```python
from build123d import *

# Parameters (mm, degrees)
SKETCH1_W           = 11.43
SKETCH1_H           = 11.43
BOSS_EXTRUDE1_DEPTH = 6.35
SKETCH3_W           = 6.389415989
SKETCH3_H           = 4.631950103
CUT_EXTRUDE1_DEPTH  = 7.62
SKETCH4_W           = 5.33014865
SKETCH4_H           = 6.972552684
CUT_EXTRUDE2_DEPTH  = 15.24
SKETCH5_W           = 14.938478928
SKETCH5_H           = 9.529491398
BOSS_EXTRUDE2_DEPTH = 6.35


with BuildPart() as part:
    # Sketch1 → Boss-Extrude1 (new body)
    with BuildSketch(Plane(origin=(0, 0, 0), x_dir=(1, 0, 0), z_dir=(0, 1, 0))):
        with Locations((5.715, 5.715)):
            Rectangle(SKETCH1_W, SKETCH1_H)
    extrude(amount=BOSS_EXTRUDE1_DEPTH)

    # Sketch3 → Cut-Extrude1 (cut)
    with BuildSketch(Plane(origin=(0, 0, -11.43), x_dir=(-1, 0, 0), z_dir=(0, 0, -1))):
        with Locations((-8.235292005, 4.034024949)):
            Rectangle(SKETCH3_W, SKETCH3_H)
    extrude(amount=-CUT_EXTRUDE1_DEPTH, mode=Mode.SUBTRACT)

    # Sketch4 → Cut-Extrude2 (cut)
    with BuildSketch(Plane(origin=(0, 1.718049897, 0), x_dir=(1, 0, 0), z_dir=(0, 1, 0))):
        with Locations((5.430693356, 5.379383443)):
            Rectangle(SKETCH4_W, SKETCH4_H)
    extrude(amount=CUT_EXTRUDE2_DEPTH, mode=Mode.SUBTRACT)

    # Sketch5 → Boss-Extrude2 (add)
    with BuildSketch(Plane(origin=(0, 6.35, 0), x_dir=(1, 0, 0), z_dir=(0, 1, 0))):
        with Locations((-4.703620433, 6.665254301)):
            Rectangle(SKETCH5_W, SKETCH5_H)
    extrude(amount=BOSS_EXTRUDE2_DEPTH)


solid = part.part
```
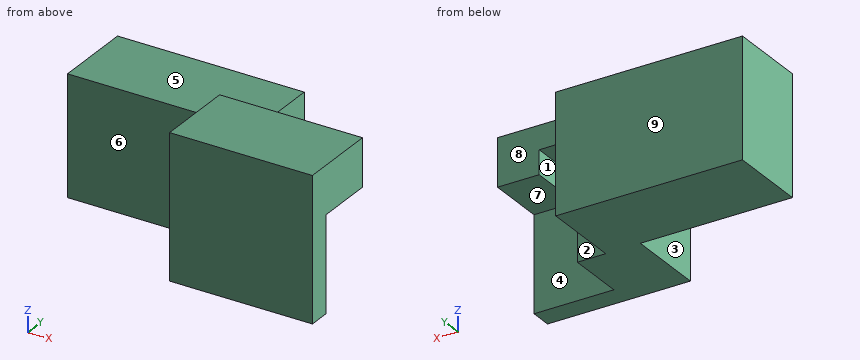
CAD build for the part. Positions are in the model's coordinates, mm. Face numbers are marked on the shaded views. A direction names the side the tool comes from. Give positions to 0.01 mm unless a question says otherwise; leave off trailing zeros. Loops run counter-clockwise (first coordinate to the right, second up) from the corner with the lowest first, then second, coordinate; pieces in that order, holes last. Notation, with made-up numbers: (44.25, 47) - (51.25, 47) arc R11 ccw to (51.25, 51) - close; hole circle Ø3 at (-7, 32). An arc over 180 degrees is marked (long way). Put each result on its own line as item: value.
Q1. Flat gauge pins, fed straight in: pin 1 (2.5 mm diameter, centred on x = 6, y = 4, fed in from -Z); pin 2 (3 mm diameter, centred on x = -2.5, z = -7, fed in from -Y); pin 3 (0.6 mm diameter, centred on y = 4.5, z = -2.5, fed in from -X); pin 4 (1.1 mm diameter, centred on x = 4, z = -10.5, fed in from +Y). Where does each tip first touch, or does it go through?
Filled in:
pin 1: stops at z = -11.43
pin 2: stops at y = 6.35
pin 3: stops at x = 0
pin 4: stops at y = 6.35
Q2. Slice it at D-D (z = -2.5). Give the cut face in (x, y).
Filled in:
outline: (-12.17, 6.35) - (0, 6.35) - (0, 0) - (11.43, 0) - (11.43, 6.35) - (8.1, 6.35) - (8.1, 1.72) - (2.77, 1.72) - (2.77, 12.7) - (-12.17, 12.7) - close
Q3. Slice it at A-A (z = -8.5). Give the cut face in (x, y), plus the area to 3 significant figures.
Filled in:
outline: (-12.17, 6.35) - (0, 6.35) - (0, 0) - (11.43, 0) - (11.43, 1.72) - (2.77, 1.72) - (2.77, 12.7) - (-12.17, 12.7) - close
area: 127 mm²
Q4. Tool access for the marked faces 5, 6, 7, 8 and 9: list every direction of +Z, -Z, +X, -X, +Y, -Y with a clear straight run to the whole face (end or side of a thin tool).
Filled in:
face 5: +Z, +X, -X, +Y
face 6: +Z, -Z, -X, -Y
face 7: -Z, +X, +Y
face 8: +Z, +X, +Y
face 9: +Z, -Z, +X, -X, +Y
Q5. Mould opens along X. For the marked faces 1, 2, 3 and 4 say: pulls with the +X half, pulls with the -X half, needs draft (parallel to the pull), parting line crosses it, or undercut.
Filled in:
face 1: undercut
face 2: needs draft
face 3: pulls with the -X half
face 4: undercut
Q6. Slice it at B-B (y = 6). Give the cut face in (x, z), plus the area to 3 significant figures.
Filled in:
outline: (0, -11.43) - (5.04, -11.43) - (5.04, -8.87) - (2.77, -8.87) - (2.77, -1.89) - (8.1, -1.89) - (8.1, -3.81) - (11.43, -3.81) - (11.43, 0) - (0, 0) - close
area: 60.2 mm²
Q7. Probe line 1 along X through (y, z) = (3.5, -3); line 2 along X through (y, z) = (2.5, -1.25); line 3 along Z through (x, y) = (-8, 8). List the from-to ranges inside material, lowest first.
Filled in:
line 1: x = 0 to 2.77, 8.1 to 11.43
line 2: x = 0 to 11.43
line 3: z = -11.43 to -1.9
Q8. Slice it at C-C (x = 5.75). Give the cut face in (y, z), plus the area to 3 significant figures.
Filled in:
outline: (0, -11.43) - (1.72, -11.43) - (1.72, -1.89) - (6.35, -1.89) - (6.35, 0) - (0, 0) - close
area: 28.4 mm²
